Check sheet for the modelled part. Datum: model origin and axes. Units: mm. Give positions to 0.01 mm unless a question says otherwise; leave off trailing zeros. Write item = value, one per line. Start each with the question number.
1) Gauge pin test, flat ends, axial feed: pin 1 (2 mm diameter, centred on y = 351.5, z = -9, fed in from +X); pin 2 (10 mm diameter, centred on x = -45, z = 64.5, fed in from +Y); pin 3 (5 mm diameter, centred on x = -19.5, y = 353, fed in from -Z). Record the tip position at first contact, or that the pin passes through.
2) Draft check along Z on faces 1 (the face through (93.36, 348.64, -29.4)), 2 (the face through (-41.71, 364.07, 52.2)), 3 (the face through (41.71, 364.07, -52.2)), 4 (the face through (34.976, 367.041, 34.289)). Enter one of: pulls with the +Z half, pulls with the -Z half, needs draft (parallel to the pull), parting line crosses it, or undercut.
3) Scan lines: L1, parallel to Y at x = 74.5, z = -12.5; L2, parallel to Y at x = 45, z = -2. Record each from-to range of solid material in increasing order.
from build123d import *

# Parameters (mm, degrees)
CUT_REVOLVE1_OUTLINE_W     = 1
CUT_REVOLVE1_OUTLINE_H     = 2.00606464
CUT_REVOLVE1_START         = -360.979129626
CUT_REVOLVE1_2_OUTLINE_R   = 2
CUT_REVOLVE1_2_OUTLINE_R_2 = 1
CUT_REVOLVE1_2_DEPTH       = 1.979129626
CUT_REVOLVE1_START_2       = -363
CUT_REVOLVE1_3_OUTLINE_R   = 1
CUT_REVOLVE1_3_DEPTH       = 0.522870482
CIRPATTERN2_COUNT          = 4
CIRPATTERN3_COUNT          = 4


with BuildPart() as part:
    # Sketch1 → Revolve1 (revolve)
    with BuildSketch(Plane.XY, mode=Mode.PRIVATE) as revolve1_sk:
        with BuildLine():
            ThreePointArc((0, 368.638544248), (-49.884385754, 363.569703341), (-97.729610096, 348.570383425))
            Line((-97.729610096, 348.570383425), (-100.153071713, 349.700462136))
            ThreePointArc((-100.153071713, 349.700462136), (-51.159165982, 365.348044955), (0, 370.638544248))
            Line((0, 370.638544248), (0, 368.638544248))
        make_face()
    revolve(revolve1_sk.sketch.rotate(Axis((0, 394.944466532, 0), (0, 1, 0)), 180), axis=Axis((0, 394.944466532, 0), (0, 1, 0)))

    # Cut-Revolve1: read off the stored shape, not the designer's step
    # Cut-Revolve1 outline → Cut-Revolve1 (revolve, cut)
    with BuildSketch(Plane(origin=(40.663332066, 15.766965619, 0), x_dir=(0.932364777994183, 0.361518907881535, 0), z_dir=(0, 0, -1))):
        with Locations((0.5, -361.474097198)):
            Rectangle(CUT_REVOLVE1_OUTLINE_W, CUT_REVOLVE1_OUTLINE_H)
    cut_revolve1 = revolve(axis=Axis((40.663332066, 15.766965619, 0), (0.361518907881535, -0.932364777994183, 0)), mode=Mode.SUBTRACT)

    # Cut-Revolve1 2 outline → Cut-Revolve1 2 (cut)
    with BuildSketch(Plane(origin=(0, 0, 0), x_dir=(0.932364777994183, 0.361518907881535, 0), z_dir=(0.361518907881535, -0.932364777994183, 0)).offset(CUT_REVOLVE1_START)):
        with Locations((43.613114765, 0)):
            Circle(CUT_REVOLVE1_2_OUTLINE_R)
        with Locations((43.613114765, 0)):
            Circle(CUT_REVOLVE1_2_OUTLINE_R_2, mode=Mode.SUBTRACT)
    cut_revolve1_2 = extrude(amount=CUT_REVOLVE1_2_DEPTH, mode=Mode.SUBTRACT)

    # Cut-Revolve1 3 outline → Cut-Revolve1 3 (cut)
    with BuildSketch(Plane(origin=(0, 0, 0), x_dir=(0.932364777994183, 0.361518907881535, 0), z_dir=(0.361518907881535, -0.932364777994183, 0)).offset(CUT_REVOLVE1_START_2)):
        with Locations((43.613114765, 0)):
            Circle(CUT_REVOLVE1_3_OUTLINE_R)
    cut_revolve1_3 = extrude(amount=CUT_REVOLVE1_3_DEPTH, mode=Mode.SUBTRACT)

    # Cut-Revolve1 4 outline → Cut-Revolve1 4 (revolve)
    with BuildSketch(Plane(origin=(40.663332066, 15.766965619, 0), x_dir=(0.932364777994183, 0.361518907881535, 0), z_dir=(0, 0, -1))):
        with BuildLine():
            ThreePointArc((2, -360.977117445), (1.500001012, -360.978626505), (1, -360.979129526))
            Line((1, -360.979129526), (2, -360.979129526))
            Line((2, -360.979129526), (2, -360.977117445))
        make_face()
    cut_revolve1_4 = revolve(axis=Axis((40.663332066, 15.766965619, 0), (0.361518907881535, -0.932364777994183, 0)))

    # CirPattern2: Cut-Revolve1, Cut-Revolve1 2, Cut-Revolve1 3, Cut-Revolve1 4 ×4 about axis
    cirpattern2_axis = Axis((0, 0, 0), (0, 1, 0))
    add([cut_revolve1.rotate(cirpattern2_axis, i * 360 / CIRPATTERN2_COUNT) for i in range(1, CIRPATTERN2_COUNT)], mode=Mode.SUBTRACT)
    add([cut_revolve1_2.rotate(cirpattern2_axis, i * 360 / CIRPATTERN2_COUNT) for i in range(1, CIRPATTERN2_COUNT)], mode=Mode.SUBTRACT)
    add([cut_revolve1_3.rotate(cirpattern2_axis, i * 360 / CIRPATTERN2_COUNT) for i in range(1, CIRPATTERN2_COUNT)], mode=Mode.SUBTRACT)
    add([cut_revolve1_4.rotate(cirpattern2_axis, i * 360 / CIRPATTERN2_COUNT) for i in range(1, CIRPATTERN2_COUNT)])

    # Sketch5 → Cut-Revolve5 (revolve, cut)
    with BuildSketch(Plane(origin=(0, 0, 0), x_dir=(0, 1, 0), z_dir=(0.7071067811865488, 0, 0.7071067811865464))):
        with BuildLine():
            Line((365.638544248, 60), (356.088544248, 60))
            ThreePointArc((356.088544248, 60), (356.157319563, 58.855937734), (356.362654922, 57.728353634))
            Line((356.362654922, 57.728353634), (365.638544248, 60))
        make_face()
        with BuildLine():
            Line((375.188544248, 60), (365.638544248, 60))
            Line((365.638544248, 60), (356.362654922, 57.728353634))
            ThreePointArc((356.362654922, 57.728353634), (359.68698401, 52.531303278), (365.495009667, 50.451078709))
            ThreePointArc((365.495009667, 50.451078709), (372.340474744, 53.196572362), (375.188544248, 60))
        make_face()
    cut_revolve5 = revolve(axis=Axis((-42.426406871, 356.088544248, 42.426406871), (0, -1, 0)), mode=Mode.SUBTRACT)

    # Sketch5_9 → Revolve3 (revolve)
    with BuildSketch(Plane(origin=(0, 0, 0), x_dir=(0, 1, 0), z_dir=(0.7071067811865488, 0, 0.7071067811865464))):
        Polygon((359.989382103, 69.993068922), (360.346185197, 68.536122954), (363.366897883, 69.275889326), (363.010094789, 70.732835294), align=None)
    revolve3 = revolve(axis=Axis((0, 120.638544248, 0), (-0.1681985915763013, 0.9712973116319725, 0.16819859157630185)))

    # CirPattern3: Cut-Revolve5, Revolve3 ×4 about axis
    cirpattern3_axis = Axis((0, 0, 0), (0, 1, 0))
    add([cut_revolve5.rotate(cirpattern3_axis, i * 360 / CIRPATTERN3_COUNT) for i in range(1, CIRPATTERN3_COUNT)], mode=Mode.SUBTRACT)
    add([revolve3.rotate(cirpattern3_axis, i * 360 / CIRPATTERN3_COUNT) for i in range(1, CIRPATTERN3_COUNT)])


solid = part.part
Data:
q1.pin_1 = 97.89
q1.pin_2 = 359.54
q1.pin_3 = -96.37
q2.face_1 = parting line crosses it
q2.face_2 = pulls with the +Z half
q2.face_3 = pulls with the -Z half
q2.face_4 = undercut
q3.L1 = 356.85 to 358.95
q3.L2 = 364.51 to 366.55
